```python
from build123d import *

# Parameters (mm, degrees)
SKETCH1_R               = 4
SKETCH1_R_2             = 2
BOSS_EXTRUDE1_DEPTH     = 5
SKETCH2_R               = 4
SKETCH2_R_2             = 2
BOSS_EXTRUDE2_DEPTH     = 5
CUT_EXTRUDE1_DEPTH      = 9.124038528
CUT_EXTRUDE1_DEPTH_BACK = 9.124038528
SKETCH1_2_R             = 2
CUT_EXTRUDE2_DEPTH      = 9.124038528
CUT_EXTRUDE2_DEPTH_BACK = 9.124038528
SKETCH2_2_R             = 2


with BuildPart() as part:
    # Sketch1 → Boss-Extrude1 (new, symmetric)
    with BuildSketch(Plane.XY):
        Circle(SKETCH1_R)
        Circle(SKETCH1_R_2, mode=Mode.SUBTRACT)
    extrude(amount=BOSS_EXTRUDE1_DEPTH, both=True)

    # Sketch2 → Boss-Extrude2 (add, symmetric)
    with BuildSketch(Plane(origin=(0, 0, 0), x_dir=(1, 0, 0), z_dir=(0, 1, 0))):
        Circle(SKETCH2_R)
        with Locations(Location((0, 0, 0), (0, 0, 90))):
            Circle(SKETCH2_R_2, mode=Mode.SUBTRACT)
    extrude(amount=BOSS_EXTRUDE2_DEPTH, both=True)

    # Sketch1_2 → Cut-Extrude1 (cut, two sides: drawn at the far end of the back side and taken through both)
    with BuildSketch(Plane.XY.offset(-CUT_EXTRUDE1_DEPTH_BACK)):
        Circle(SKETCH1_2_R)
    extrude(amount=CUT_EXTRUDE1_DEPTH + CUT_EXTRUDE1_DEPTH_BACK, mode=Mode.SUBTRACT)

    # Sketch2_2 → Cut-Extrude2 (cut, two sides: drawn at the far end of the back side and taken through both)
    with BuildSketch(Plane(origin=(0, 0, 0), x_dir=(1, 0, 0), z_dir=(0, 1, 0)).offset(-CUT_EXTRUDE2_DEPTH_BACK)):
        with Locations(Location((0, 0, 0), (0, 0, 180))):
            Circle(SKETCH2_2_R)
    extrude(amount=CUT_EXTRUDE2_DEPTH + CUT_EXTRUDE2_DEPTH_BACK, mode=Mode.SUBTRACT)


solid = part.part
```
Build history of the part. All positions in model axes, mm. A direction names the side the tool comes from. Coordinates: 2 decimals unless noted, no trailing zeros. Write each loop counter-clockwise with the first axis right and the second up, starting at its lowest first coordinate (ties: lowest second). Pieces come first, ordered by that corner, then holes.
1. Band-saw the part on C-C, the plane y = -2.5. Give the cut face in (x, z), and give its area (3 significant figures).
Answer block:
outline: (-3.12, -5) - (3.12, -5) - (3.12, -2.5) arc R4 ccw to (3.12, 2.5) - (3.12, 5) - (-3.12, 5) - (-3.12, 2.5) arc R4 ccw to (-3.12, -2.5) - close; hole circle Ø4 at (0, 0)
area: 55.9 mm2
2. Drill centre lines: probe 1 along Y at (x, z) = (0, -4.2); probe 2 along Y at (x, z) = (0, -2.9). Where is each one in solid material? Low to high.
Answer block:
probe 1: y = -4 to -2, 2 to 4
probe 2: y = -5 to -2, 2 to 5
3. 3-axis set-ups, long thin cutter, end or side, ignore diameter. For faces 1 (the cylindrical face through (-4, 0, 4)), 2 (the cylindrical face through (-4, -4, 0)), 3 (the cylindrical face through (-4, 0, -4)): which of +Z, -Z, +X, -X, +Y, -Y reach the whole face in a straight line?
Answer block:
face 1: +Z
face 2: -Y
face 3: -Z
4. Band-saw the part on B-B, the plane z = 0.25. Give the cut face in (x, y), and give its area (3 significant figures).
Answer block:
outline: (-3.99, -5) - (-1.98, -5) - (-1.98, -0.25) arc R2 cw to (-1.98, 0.25) - (-1.98, 5) - (-3.99, 5) - (-3.99, 0.25) arc R4 ccw to (-3.99, -0.25) - close; (1.98, -5) - (3.99, -5) - (3.99, -0.25) arc R4 ccw to (3.99, 0.25) - (3.99, 5) - (1.98, 5) - (1.98, 0.25) arc R2 cw to (1.98, -0.25) - close
area: 40.2 mm2
5. Drop flat-ended pins along their axis: pin 1 (3.5 mm diameter, centred on x = 0, z = 0, fed in from +Y); pin 2 (1 mm diameter, centred on x = -3, z = -3.5, fed in from +Y); pin 3 (6 mm diameter, centred on y = -3.5, z = -3.5, fed in from -X). Give the stop position or say it passes through.
Answer block:
pin 1: passes through
pin 2: stops at y = 3.12
pin 3: stops at x = -3.97
6. Band-saw the part on D-D, the plane z = 2.75. Give the cut face in (x, y), and give its area (3 significant figures).
Answer block:
outline: (-2.9, -5) - (2.9, -5) - (2.9, -2.75) arc R4 ccw to (2.9, 2.75) - (2.9, 5) - (-2.9, 5) - (-2.9, 2.75) arc R4 ccw to (-2.9, -2.75) - close; hole circle Ø4 at (0, 0)
area: 53.8 mm2
7. Band-saw the part on A-A, the plane x = 0. Give the cut face in (y, z), and give its area (3 significant figures).
Answer block:
outline: (-5, -4) - (-4, -4) - (-4, -5) - (-2, -5) - (-2, -2) - (-5, -2) - close; (-5, 2) - (-2, 2) - (-2, 5) - (-4, 5) - (-4, 4) - (-5, 4) - close; (2, -5) - (4, -5) - (4, -4) - (5, -4) - (5, -2) - (2, -2) - close; (2, 2) - (5, 2) - (5, 4) - (4, 4) - (4, 5) - (2, 5) - close
area: 32.0 mm2
